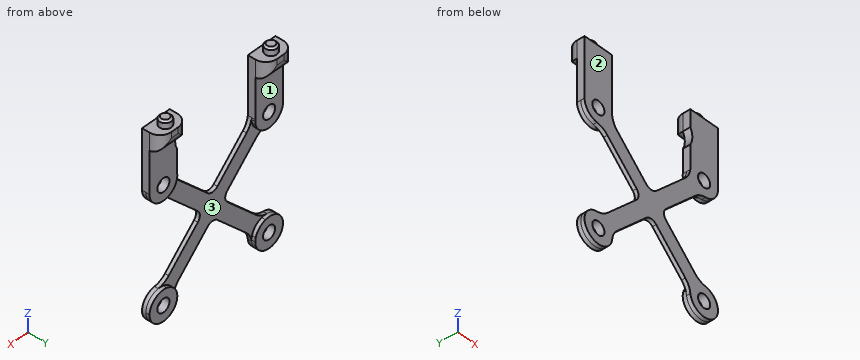
from build123d import *

# Parameters (mm, degrees)
SKETCH1_R           = 1.75
BOSS_EXTRUDE1_DEPTH = 1
SKETCH2_R           = 1.75
BOSS_EXTRUDE2_DEPTH = 1
FILLET1_R           = 5
FILLET2_R           = 2
BOSS_EXTRUDE3_REACH = 29.297
CUT_EXTRUDE1_REACH  = 38.486
SKETCH4_R           = 4.38
SKETCH5_W           = 7.977665541
SKETCH5_H           = 4.558516631
BOSS_EXTRUDE4_DEPTH = 3
SKETCH6_R           = 1.55
BOSS_EXTRUDE5_DEPTH = 2
FILLET3_R           = 3
CHAMFER1_SIZE       = 0.5


# Some blends are built 0.0001 mm under size
with BuildPart() as part:
    # Sketch1 → Boss-Extrude1 (new body)
    with BuildSketch(Plane(origin=(0, 0, 0), x_dir=(1, 0, 0), z_dir=(0, 1, 0))):
        with BuildLine():
            ThreePointArc((-11.386296695, 14.21472382), (-18.078427125, 18.078427125), (-14.21472382, 11.386296695))
            Line((-14.21472382, 11.386296695), (-2.828427125, 0))
            Line((-2.828427125, 0), (-14.21472382, -11.386296695))
            ThreePointArc((-14.21472382, -11.386296695), (-18.078427125, -18.078427125), (-11.386296695, -14.21472382))
            Line((-11.386296695, -14.21472382), (0, -2.828427125))
            Line((0, -2.828427125), (11.386296695, -14.21472382))
            ThreePointArc((11.386296695, -14.21472382), (18.078427125, -18.078427125), (14.21472382, -11.386296695))
            Line((14.21472382, -11.386296695), (2.828427125, 0))
            Line((2.828427125, 0), (14.21472382, 11.386296695))
            ThreePointArc((14.21472382, 11.386296695), (18.078427125, 18.078427125), (11.386296695, 14.21472382))
            Line((11.386296695, 14.21472382), (0, 2.828427125))
            Line((0, 2.828427125), (-11.386296695, 14.21472382))
        make_face()
        with Locations(Location((-15.25, -15.25, 0), (0, 0, 270))):
            Circle(SKETCH1_R, mode=Mode.SUBTRACT)
        with Locations(Location((15.25, -15.25, 0), (0, 0, 270))):
            Circle(SKETCH1_R, mode=Mode.SUBTRACT)
        with Locations(Location((-15.25, 15.25, 0), (0, 0, 270))):
            Circle(SKETCH1_R, mode=Mode.SUBTRACT)
        with Locations(Location((15.25, 15.25, 0), (0, 0, 270))):
            Circle(SKETCH1_R, mode=Mode.SUBTRACT)
    extrude(amount=BOSS_EXTRUDE1_DEPTH)

    # Sketch2 → Boss-Extrude2 (add)
    # profile 1 of 4: a face of its own
    with BuildSketch(Plane(origin=(0, 1, 0), x_dir=(1, 0, 0), z_dir=(0, 1, 0))):
        with BuildLine():
            ThreePointArc((-11.386296695, 14.21472382), (-11.284220555, 14.727895231), (-11.25, 15.25))
            ThreePointArc((-11.25, 15.25), (-18.423413361, 17.685045716), (-14.21472382, 11.386296695))
            ThreePointArc((-14.21472382, 11.386296695), (-12.421572875, 12.421572875), (-11.386296695, 14.21472382))
        make_face()
        with Locations(Location((-15.25, 15.25, 0), (0, 0, 270))):
            Circle(SKETCH2_R, mode=Mode.SUBTRACT)
    # profile 2 of 4: a face of its own
    with BuildSketch(Plane(origin=(0, 1, 0), x_dir=(1, 0, 0), z_dir=(0, 1, 0))):
        with BuildLine():
            ThreePointArc((-14.21472382, -11.386296695), (-18.423413361, -17.685045716), (-11.25, -15.25))
            ThreePointArc((-11.25, -15.25), (-11.284220555, -14.727895231), (-11.386296695, -14.21472382))
            ThreePointArc((-11.386296695, -14.21472382), (-12.421572875, -12.421572875), (-14.21472382, -11.386296695))
        make_face()
        with Locations(Location((-15.25, -15.25, 0), (0, 0, 270))):
            Circle(SKETCH2_R, mode=Mode.SUBTRACT)
    # profile 3 of 4: a face of its own
    with BuildSketch(Plane(origin=(0, 1, 0), x_dir=(1, 0, 0), z_dir=(0, 1, 0))):
        with BuildLine():
            ThreePointArc((11.386296695, -14.21472382), (14.727895231, -19.215779445), (19.25, -15.25))
            ThreePointArc((19.25, -15.25), (17.685045716, -12.076586639), (14.21472382, -11.386296695))
            ThreePointArc((14.21472382, -11.386296695), (12.421572875, -12.421572875), (11.386296695, -14.21472382))
        make_face()
        with Locations(Location((15.25, -15.25, 0), (0, 0, 270))):
            Circle(SKETCH2_R, mode=Mode.SUBTRACT)
    # profile 4 of 4: a face of its own
    with BuildSketch(Plane(origin=(0, 1, 0), x_dir=(1, 0, 0), z_dir=(0, 1, 0))):
        with BuildLine():
            ThreePointArc((14.21472382, 11.386296695), (17.685045716, 12.076586639), (19.25, 15.25))
            ThreePointArc((19.25, 15.25), (14.727895231, 19.215779445), (11.386296695, 14.21472382))
            ThreePointArc((11.386296695, 14.21472382), (12.421572875, 12.421572875), (14.21472382, 11.386296695))
        make_face()
        with Locations(Location((15.25, 15.25, 0), (0, 0, 270))):
            Circle(SKETCH2_R, mode=Mode.SUBTRACT)
    extrude(amount=BOSS_EXTRUDE2_DEPTH)

    # Fillet1
    # the kernel refuses this fillet: 5 mm, written as the material it adds along each edge
    with BuildSketch(Plane(origin=(-11.386296695, 0, -14.21472382), x_dir=(0.07795833957339635, 0, -0.9969566175571327), z_dir=(0, 1, 0))) as fillet1_piece_1:
        with BuildLine():
            CenterArc((2.375482021, -4.915816238), FILLET1_R, 100.528779366, 38.942441269)
            Line((-1.424916256, -1.666666667), (-1.500924222, -1.601683675))
            Line((-1.500924222, -1.601683675), (-0.076007966, 0.064982991))
            Line((-0.076007966, 0.064982991), (0.018272939, 0.098316325))
            ThreePointArc((0.018272939, 0.098316325), (0.730917545, 0.03265299), (1.443562151, 0.098316325))
            Line((1.443562151, 0.098316325), (1.46183509, 0))
        make_face()
    extrude(amount=1)
    with BuildSketch(Plane(origin=(11.386296695, 0, -14.21472382), x_dir=(-0.7071067811865598, 0, 0.7071067811865355), z_dir=(0, 1, 0))) as fillet1_piece_2:
        with BuildLine():
            CenterArc((2.192752634, -5), FILLET1_R, 90, 38.942441269)
            Line((-0.949944171, -1.111111111), (-1.012798107, -1.033333333))
            ThreePointArc((-1.012798107, -1.033333333), (-0.499790959, -0.534336666), (-0.08660254, 0.05))
            Line((-0.08660254, 0.05), (0, 0.1))
            Line((0, 0.1), (2.192752634, 0.1))
            Line((2.192752634, 0.1), (2.192752634, 0))
        make_face()
    extrude(amount=1)
    with BuildSketch(Plane(origin=(14.21472382, 0, -11.386296695), x_dir=(-0.7071067811865354, 0, 0.7071067811865597), z_dir=(0, 1, 0)), Plane(origin=(11.386296695, 0, 14.21472382), x_dir=(-0.7071067811865589, 0, -0.7071067811865362), z_dir=(0, 1, 0)), Plane(origin=(-14.21472382, 0, 11.386296695), x_dir=(0.707106781186535, 0, -0.7071067811865601), z_dir=(0, 1, 0))) as fillet1_piece_3:
        with BuildLine():
            CenterArc((2.192752634, 5), FILLET1_R, 231.057558731, 38.942441269)
            Line((-0.949944171, 1.111111111), (-1.012798107, 1.033333333))
            ThreePointArc((-1.012798107, 1.033333333), (-0.499790959, 0.534336666), (-0.08660254, -0.05))
            Line((-0.08660254, -0.05), (0, -0.1))
            Line((0, -0.1), (2.192752634, -0.1))
            Line((2.192752634, -0.1), (2.192752634, 0))
        make_face()
    extrude(amount=1)
    with BuildSketch(Plane(origin=(14.21472382, 0, 11.386296695), x_dir=(0.9969566175571322, 0, -0.07795833957340413), z_dir=(0, 1, 0)), Plane(origin=(-11.386296695, 0, 14.21472382), x_dir=(0.07795833957339876, 0, 0.9969566175571326), z_dir=(0, 1, 0)), Plane(origin=(-14.21472382, 0, -11.386296695), x_dir=(-0.9969566175571319, 0, 0.07795833957340663), z_dir=(0, 1, 0))) as fillet1_piece_4:
        with BuildLine():
            CenterArc((2.375482021, 4.915816238), FILLET1_R, 220.528779366, 38.942441269)
            Line((-1.424916256, 1.666666667), (-1.500924222, 1.601683675))
            Line((-1.500924222, 1.601683675), (-0.076007966, -0.064982991))
            Line((-0.076007966, -0.064982991), (0.018272939, -0.098316325))
            ThreePointArc((0.018272939, -0.098316325), (0.730917545, -0.03265299), (1.443562151, -0.098316325))
            Line((1.443562151, -0.098316325), (1.46183509, 0))
        make_face()
    extrude(amount=1)

    # Fillet2
    fillet2_edges = [part.edges().sort_by_distance(p)[0] for p in [
        (0, 0.5, -2.828427125),
        (2.828427125, 0.5, 0),
        (0, 0.5, 2.828427125),
        (-2.828427125, 0.5, 0),
    ]]
    fillet(fillet2_edges, radius=FILLET2_R)

    # Boss-Extrude3: up to this face of the body (flat: up to its plane)
    boss_extrude3_end = Plane(part.part.faces().sort_by_distance((11.363137085, 2, 15.25))[0])
    # Sketch3 → Boss-Extrude3 (add, up to the picked face)
    with BuildSketch(Plane.XZ, mode=Mode.PRIVATE) as boss_extrude3_sk1:
        with BuildLine():
            Line((-11.272334459, 30.93), (-19.25, 30.93))
            Line((-19.25, 30.93), (-19.25, 15.25))
            ThreePointArc((-19.25, 15.25), (-15.461350224, 19.244412483), (-11.272334459, 15.672109986))
            Line((-11.272334459, 15.672109986), (-11.272334459, 30.93))
        make_face()
    boss_extrude3_tool1 = split(extrude(boss_extrude3_sk1.sketch, amount=-BOSS_EXTRUDE3_REACH, mode=Mode.PRIVATE), bisect_by=boss_extrude3_end, keep=Keep.BOTH, mode=Mode.PRIVATE)
    # Sketch3 → Boss-Extrude3 (add, up to the picked face)
    with BuildSketch(Plane.XZ, mode=Mode.PRIVATE) as boss_extrude3_sk2:
        with BuildLine():
            Line((19.25, 30.93), (11.272334459, 30.93))
            Line((11.272334459, 30.93), (11.272334459, 15.672109986))
            ThreePointArc((11.272334459, 15.672109986), (15.461350224, 19.244412483), (19.25, 15.25))
            Line((19.25, 15.25), (19.25, 30.93))
        make_face()
    boss_extrude3_tool2 = split(extrude(boss_extrude3_sk2.sketch, amount=-BOSS_EXTRUDE3_REACH, mode=Mode.PRIVATE), bisect_by=boss_extrude3_end, keep=Keep.BOTH, mode=Mode.PRIVATE)
    add(boss_extrude3_tool1.solids().sort_by(Axis((-15.263723, 0, 24.633823), (0, 1, 0)))[0])
    add(boss_extrude3_tool2.solids().sort_by(Axis((15.263723, 0, 24.633823), (0, 1, 0)))[0])

    # Sketch4 → Cut-Extrude1 (cut, up to next)
    with BuildSketch(Plane(origin=(0, 2, 0), x_dir=(1, 0, 0), z_dir=(0, 1, 0)), mode=Mode.PRIVATE) as cut_extrude1_sk1:
        with Locations((7.48, -24.18)):
            Circle(SKETCH4_R)
    cut_extrude1_tool1 = extrude(cut_extrude1_sk1.sketch, amount=-CUT_EXTRUDE1_REACH, mode=Mode.PRIVATE) & part.part
    add(cut_extrude1_tool1.solids().sort_by_distance((7.48, 2, 24.18))[0], mode=Mode.SUBTRACT)

    # Sketch5 → Boss-Extrude4 (add)
    with BuildSketch(Plane(origin=(0, 2, 0), x_dir=(1, 0, 0), z_dir=(0, 1, 0))):
        with Locations((-15.261167229, -28.650741685)):
            Rectangle(SKETCH5_W, SKETCH5_H)
        with Locations((15.261167229, -28.650741685)):
            Rectangle(SKETCH5_W, SKETCH5_H)
    extrude(amount=BOSS_EXTRUDE4_DEPTH)

    # Sketch6 → Boss-Extrude5 (add)
    with BuildSketch(Plane.XY.offset(30.93)):
        with Locations(Location((-15.25, 2.5, 0), (0, 0, 180))):
            Circle(SKETCH6_R)
        with Locations(Location((15.25, 2.5, 0), (0, 0, 180))):
            Circle(SKETCH6_R)
    extrude(amount=BOSS_EXTRUDE5_DEPTH)

    # Fillet3
    fillet3_edges = [part.edges().sort_by_distance(p)[0] for p in [
        (19.25, 5, 28.650741684),
        (11.272334459, 5, 28.650741684),
        (-11.272334459, 5, 28.650741684),
        (-19.25, 5, 28.650741684),
        (15.261167229, 5, 26.371483369),
        (-15.261167229, 5, 26.371483369),
    ]]
    fillet(fillet3_edges, radius=FILLET3_R - 0.0001)  # a hair under: the kernel refuses the full size

    # Chamfer1
    chamfer1_edges = [part.edges().sort_by_distance(p)[0] for p in [
        (-13.7, 2.5, 32.93),
        (16.8, 2.5, 32.93),
    ]]
    chamfer(chamfer1_edges, length=CHAMFER1_SIZE)


solid = part.part
For this review, take the finished solid that the model builds, in its own axes (mm). Face numbers are marked on the shaded views. A direction names the side the tool comes from. Give positions to 0.01 mm unless a question says otherwise; leave off trailing zeros. Loops run counter-clockwise (first coordinate to the right, second up) from the corner with the lowest first, then second, coordinate; pieces in that order, holes last.
Item 1: Take a section at A-A, the plane x = -10.5. State the section outline as (y, z) points.
Item 2: Take a section at B-B, the plane z = -5. State the section outline as (x, y) points.
Item 3: For line 1 along X through (y, z) = (1.55, -15.25); line 2 along Z through (x, y) = (-14, 1.15); line 3 along X through (y, z) = (0.6, 15.25), list the stretches that pass through material, from the lowest coordinate up.
Item 4: Take a section at C-C, the plane x = -2.5. State the section outline as (y, z) points, and give its area (3 significant figures).
Item 5: Insertion check: pin 1 (2 mm diameter, centred on x = -15.25, z = -15.25, fed in from -Y); pin 2 (6.5 mm diameter, centred on x = -16.5, z = 17, fed in from +Y); pin 3 (9.5 mm diameter, centred on x = -7.5, z = -8, fed in from +Y); pin 4 (2 mm diameter, centred on x = 14, y = 2, fed in from -Z). Each pin has a flat end and moves straight along its axis. Give the tip position at first contact, or say it passes through.
Item 6: Tool access review of the marked faces 1, 2 and 3: name each direction out of +Z, -Z, +X, -X, +Y, -Y from which nothing blocks a thin tool from reaching the whole face with its end or side.
Calculated:
1. outline: (0, -13.49) - (1, -13.49) - (1, -7.67) - (0, -7.67) - close; (0, 7.67) - (1, 7.67) - (1, 13.49) - (0, 13.49) - close
2. outline: (-7.83, 0) - (-2.17, 0) - (-2.17, 1) - (-7.83, 1) - close; (2.17, 0) - (7.83, 0) - (7.83, 1) - (2.17, 1) - close
3. line 1: x = -19.25 to -17, -13.5 to -11.25, 11.25 to 13.5, 17 to 19.25
3. line 2: z = -19.05 to -16.47, -14.03 to -11.45, 11.45 to 14.03, 16.47 to 30.93
3. line 3: x = -19.25 to -17, -13.5 to -11.21, 11.21 to 13.5, 17 to 19.25
4. outline: (0, -5.33) - (1, -5.33) - (1, 5.33) - (0, 5.33) - close
4. area: 10.7 mm2
5. pin 1: passes through
5. pin 2: stops at y = 2
5. pin 3: stops at y = 1
5. pin 4: stops at z = -19.24
6. face 1: -Z, +X, -X, +Y
6. face 2: +Z, -Z, +X, -X, -Y
6. face 3: +Y
